from build123d import *

# Parameters (mm, degrees)
F0_W     = 25.4
F0_H     = 25.4
F1_DEPTH = 444.5
F2_R     = 6.35
F3_DEPTH = 25.401
F4_R     = 6.35
F5_DEPTH = 25.401


with BuildPart() as f1:
    # F0 (on Front) → F1 (new body, symmetric)
    with BuildSketch(Plane.XZ):
        Rectangle(F0_W, F0_H)
    extrude(amount=F1_DEPTH, both=True)

    # F2 (on face) → F3 (cut, through all)
    with BuildSketch(Plane.YZ.offset(12.7)):
        with Locations((-431.8, 0)):
            Circle(F2_R)
        with Locations((431.8, 0)):
            Circle(F2_R)
    extrude(amount=-F3_DEPTH, mode=Mode.SUBTRACT)

    # F4 (on face) → F5 (cut, through all)
    with BuildSketch(Plane.YZ.offset(12.7)):
        Circle(F4_R)
    extrude(amount=-F5_DEPTH, mode=Mode.SUBTRACT)


solid = f1.part
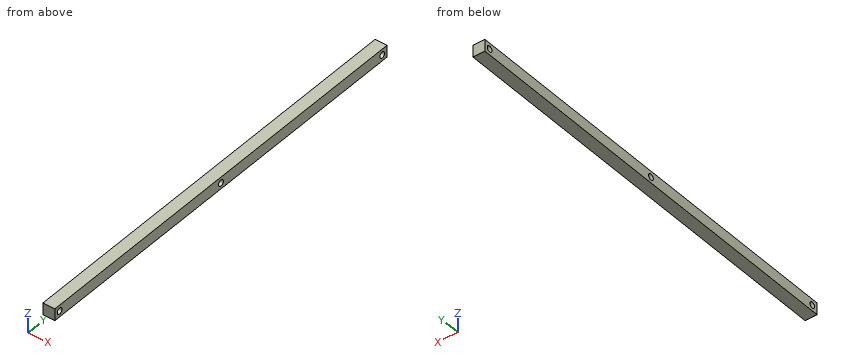
Geometry: final body of the model. Coordinates: model frame, mm. Give positions to 0.01 mm unless a question says otherwise; leave off trailing zeros. Write each loop counter-clockwise with the first axis right and the second up, starting at its lowest first coordinate (ties: lowest second). Pieces come first, ordered by that corner, then holes. Notation, with made-up numbers: (69, 44) -> (86, 44) arc R12 ccw to (86, 57) -> close; hole circle Ø10 at (-21, 81.25). An arc over 180 degrees is marked (long way). Answer in a Markdown table with one row per item.
(1) Section query B-B on x = 5.5. Return loops of the section in (y, z).
Answers below:
| item | result |
|---|---|
| outline | (-444.5, -12.7) -> (444.5, -12.7) -> (444.5, 12.7) -> (-444.5, 12.7) -> close; hole circle Ø12.7 at (-431.8, 0); hole circle Ø12.7 at (0, 0); hole circle Ø12.7 at (431.8, 0) |
(2) Pin query (flat end, axial travel): pin 1 (14.5 mm diameter, centred on y = 431.8, z = 0, fed in from +X). Return the tip coordinate at first contact, or that it passes through.
Answers below:
| item | result |
|---|---|
| pin 1 | x = 12.7 |
(3) Ray query, line 1 along Y through (x, z) = (-3.75, -1); line 2 along Z through (x, y) = (2.5, 431.8); line 3 along Y through (x, z) = (-0.25, 5). Return the intervals inside material, ascending. Write a range as [from, to].
Answers below:
| item | result |
|---|---|
| line 1 | [-444.5, -438.07], [-425.53, -6.27], [6.27, 425.53], [438.07, 444.5] |
| line 2 | [-12.7, -6.35], [6.35, 12.7] |
| line 3 | [-444.5, -435.71], [-427.89, -3.91], [3.91, 427.89], [435.71, 444.5] |
(4) Section query A-A on z = 0. Return loops of the section in (x, y), then the cut area to 3 significant figures.
Answers below:
| item | result |
|---|---|
| outline | (-12.7, -444.5) -> (12.7, -444.5) -> (12.7, -438.15) -> (-12.7, -438.15) -> close; (-12.7, -425.45) -> (12.7, -425.45) -> (12.7, -6.35) -> (-12.7, -6.35) -> close; (-12.7, 6.35) -> (12.7, 6.35) -> (12.7, 425.45) -> (-12.7, 425.45) -> close; (-12.7, 438.15) -> (12.7, 438.15) -> (12.7, 444.5) -> (-12.7, 444.5) -> close |
| area | 21,600 mm^2 |
